Check sheet for the drawn part. Datum: minimum x, y, z corner. Units: mm. Round coordinates to 2 decimals unless told otherwise and drop trailing zeros. Write each loop counter-clockwise with the first axis right and the second up, starting at its lowest first coordinate (ties: lowest second). Pieces come first, ordered by that corner, then holes.
Item 1: Cross-section at A-A on z = 73.57. Enter the section's corners in (x, y).
Item 2: Go/stop test with a flat-tipped pin: pin 1 Ø24 at (x, z) = (165, 50) entering from -Y. Record where the tip stops, or that it passes through.
Item 3: Material ranges on line 1 (Z direction, x = 68.57, y = 5.25); line 2 (X direction, y = 3.5, z = 26.43); line 3 (Z direction, x = 45, y = 5), recorded low to high.
Item 4: Cross-section at B-B on x = 21.43. Enter the section's corners in (y, z).
Item 5: Cross-section at C-C on x = 45. Enter the section's corners in (y, z), plus the area to 3 significant figures.
Item 6: Cross-section at D-D on y = 4.5. Count the separate pieces of the cut face and the enclosed holes in it, plus the area to 3 significant figures.
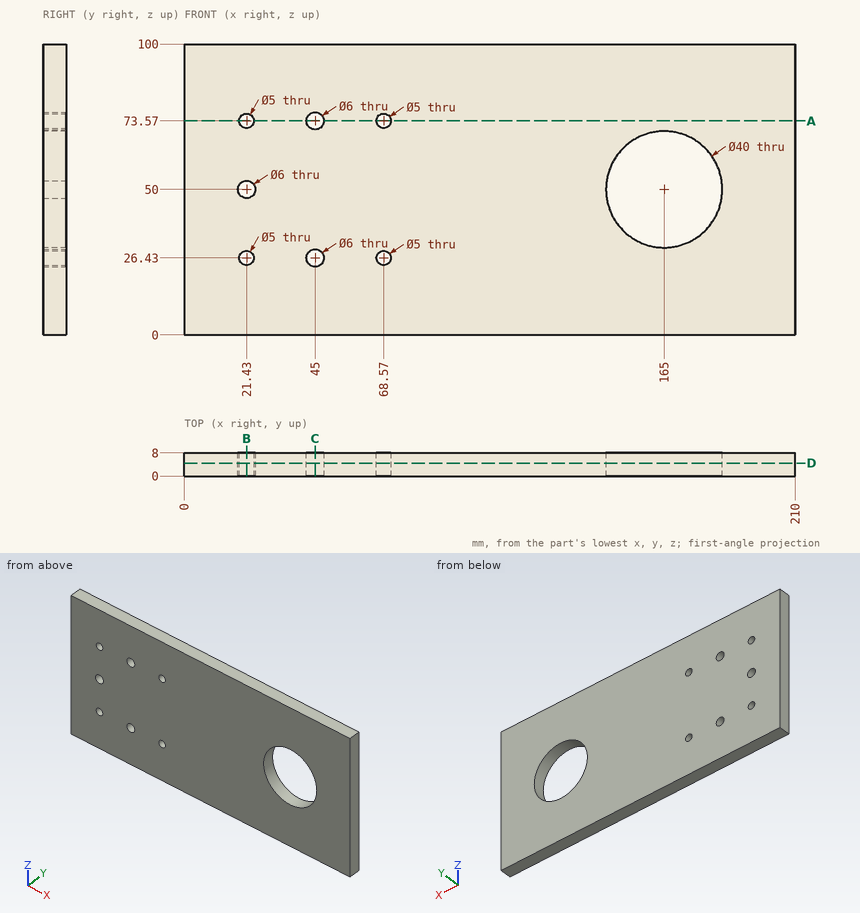
Response values:
1. outline: (0, 0) - (18.93, 0) - (18.93, 8) - (0, 8) - close; (23.93, 0) - (42, 0) - (42, 8) - (23.93, 8) - close; (48, 0) - (66.07, 0) - (66.07, 8) - (48, 8) - close; (71.07, 0) - (210, 0) - (210, 8) - (71.07, 8) - close
2. pin 1: passes through
3. line 1: z = 0 to 23.93, 28.93 to 71.07, 76.07 to 100
3. line 2: x = 0 to 18.93, 23.93 to 42, 48 to 66.07, 71.07 to 210
3. line 3: z = 0 to 23.43, 29.43 to 70.57, 76.57 to 100
4. outline: (0, 0) - (8, 0) - (8, 23.93) - (0, 23.93) - close; (0, 28.93) - (8, 28.93) - (8, 47) - (0, 47) - close; (0, 53) - (8, 53) - (8, 71.07) - (0, 71.07) - close; (0, 76.07) - (8, 76.07) - (8, 100) - (0, 100) - close
5. outline: (0, 0) - (8, 0) - (8, 23.43) - (0, 23.43) - close; (0, 29.43) - (8, 29.43) - (8, 70.57) - (0, 70.57) - close; (0, 76.57) - (8, 76.57) - (8, 100) - (0, 100) - close
5. area: 704 mm2
6. separate pieces: 1
6. enclosed holes: 8
6. area: 19,600 mm2
